```python
from build123d import *

# Parameters (mm, degrees)
F0_W     = 39.75
F0_H     = 5
F0_W_2   = 4
F0_H_2   = 9
F0_H_3   = 77
F0_W_3   = 3
F0_H_4   = 26.5
F0_H_5   = 1.95
F0_W_4   = 5
F0_H_6   = 17
F0_H_7   = 23.1
F1_DEPTH = 8


with BuildPart() as f1:
    # F0 (on Top) → F1 (new body)
    with BuildSketch(Plane.XY):
        Polygon((-32.4509056807, -49.8260023594), (-32.4509056807, -58.8260023594), (7.2990943193, -58.8260023594), (7.2990943193, -49.8260023594), (-26.0348562151, -49.8260023594), align=None)
        with Locations((-12.5759056807, -61.3260023594)):
            Rectangle(F0_W, F0_H)
        with Locations((9.2990943193, -54.3260023594)):
            Rectangle(F0_W_2, F0_H_2)
        Polygon((11.2990943193, -58.8260023594), (7.2990943193, -58.8260023594), (7.2990943193, -63.8260023594), (14.2990943193, -63.8260023594), (19.2990943193, -63.8260023594), (58.2990943193, -63.8260023594), (58.2990943193, -22.3260023594), (53.2990943193, -22.3260023594), (53.2990943193, -25.3760023594), (53.2990943193, -27.3260023594), (51.3490943193, -27.3260023594), (28.5490943193, -27.3260023594), (23.2990943193, -27.3260023594), (23.2990943193, -32.3260023594), (53.5990943193, -32.3260023594), (55.2990943193, -32.3260023594), (55.2990943193, -34.0260023594), (55.2990943193, -57.1260023594), (55.2990943193, -58.8260023594), (53.5990943193, -58.8260023594), (23.2990943193, -58.8260023594), (19.2990943193, -58.8260023594), (14.2990943193, -58.8260023594), align=None)
        with BuildLine():
            Line((-32.4509056807, -0.3260023594), (-32.4509056807, -49.8260023594))
            Line((-32.4509056807, -49.8260023594), (-26.0348562151, -49.8260023594))
            Line((-26.0348562151, -49.8260023594), (7.2990943193, -49.8260023594))
            Line((7.2990943193, -49.8260023594), (11.2990943193, -49.8260023594))
            Line((11.2990943193, -49.8260023594), (11.2990943193, -49.2260023594))
            ThreePointArc((11.2990943193, -49.2260023594), (9.2990943193, -47.2260023594), (11.2990943193, -45.2260023594))
            Line((11.2990943193, -45.2260023594), (11.2990943193, -0.3260023594))
            Line((11.2990943193, -0.3260023594), (-32.4509056807, -0.3260023594))
        make_face()
        with Locations((-12.5759056807, -102.3260023594)):
            Rectangle(F0_W, F0_H_3)
        with Locations((12.7990943193, -54.3260023594)):
            Rectangle(F0_W_3, F0_H_2)
        Polygon((14.2990943193, -49.8260023594), (14.2990943193, -58.8260023594), (19.2990943193, -58.8260023594), (19.2990943193, -32.3260023594), (23.2990943193, -32.3260023594), (23.2990943193, -27.3260023594), (19.2990943193, -27.3260023594), (19.2990943193, -25.3760023594), (19.2990943193, -2.2760023594), (19.2990943193, -0.3260023594), (14.2990943193, -0.3260023594), (14.2990943193, -27.3260023594), (14.2990943193, -32.3260023594), (14.2990943193, -47.2260023594), align=None)
        with BuildLine():
            Line((11.2990943193, -49.2260023594), (11.2990943193, -49.8260023594))
            Line((11.2990943193, -49.8260023594), (14.2990943193, -49.8260023594))
            Line((14.2990943193, -49.8260023594), (14.2990943193, -47.2260023594))
            Line((14.2990943193, -47.2260023594), (13.2990943193, -47.2260023594))
            ThreePointArc((13.2990943193, -47.2260023594), (12.7133078817, -48.6402159218), (11.2990943193, -49.2260023594))
        make_face()
        with BuildLine():
            Line((14.2990943193, -0.3260023594), (11.2990943193, -0.3260023594))
            Line((11.2990943193, -0.3260023594), (11.2990943193, -45.2260023594))
            ThreePointArc((11.2990943193, -45.2260023594), (12.7133078817, -45.811788797), (13.2990943193, -47.2260023594))
            Line((13.2990943193, -47.2260023594), (14.2990943193, -47.2260023594))
            Line((14.2990943193, -47.2260023594), (14.2990943193, -32.3260023594))
            Line((14.2990943193, -32.3260023594), (14.2990943193, -27.3260023594))
            Line((14.2990943193, -27.3260023594), (14.2990943193, -0.3260023594))
        make_face()
        with Locations((21.2990943193, -45.5760023594)):
            Rectangle(F0_W_2, F0_H_4)
        with BuildLine():
            Line((23.2990943193, -32.3260023594), (23.2990943193, -58.8260023594))
            Line((23.2990943193, -58.8260023594), (53.5990943193, -58.8260023594))
            Line((53.5990943193, -58.8260023594), (53.5990943193, -58.3260023594))
            ThreePointArc((53.5990943193, -58.3260023594), (52.7505661819, -56.277474222), (54.7990943193, -57.1260023594))
            Line((54.7990943193, -57.1260023594), (55.2990943193, -57.1260023594))
            Line((55.2990943193, -57.1260023594), (55.2990943193, -34.0260023594))
            Line((55.2990943193, -34.0260023594), (54.7990943193, -34.0260023594))
            ThreePointArc((54.7990943193, -34.0260023594), (52.7505661819, -34.8745304968), (53.5990943193, -32.8260023594))
            Line((53.5990943193, -32.8260023594), (53.5990943193, -32.3260023594))
            Line((53.5990943193, -32.3260023594), (23.2990943193, -32.3260023594))
        make_face()
        with Locations((21.2990943193, -1.3010023594)):
            Rectangle(F0_W_2, F0_H_5)
        with BuildLine():
            Line((53.5990943193, -58.3260023594), (53.5990943193, -58.8260023594))
            Line((53.5990943193, -58.8260023594), (55.2990943193, -58.8260023594))
            Line((55.2990943193, -58.8260023594), (55.2990943193, -57.1260023594))
            Line((55.2990943193, -57.1260023594), (54.7990943193, -57.1260023594))
            ThreePointArc((54.7990943193, -57.1260023594), (54.4476224568, -57.9745304968), (53.5990943193, -58.3260023594))
        make_face()
        with Locations((55.7990943193, -13.8260023594)):
            Rectangle(F0_W_4, F0_H_6)
        with BuildLine():
            Line((28.5490943193, -0.3260023594), (23.2990943193, -0.3260023594))
            Line((23.2990943193, -0.3260023594), (23.2990943193, -2.2760023594))
            Line((23.2990943193, -2.2760023594), (27.3990943193, -2.2760023594))
            ThreePointArc((27.3990943193, -2.2760023594), (27.735921521, -1.462829561), (28.5490943193, -1.1260023594))
            Line((28.5490943193, -1.1260023594), (28.5490943193, -0.3260023594))
        make_face()
        with Locations((21.2990943193, -13.8260023594)):
            Rectangle(F0_W_2, F0_H_7)
        with BuildLine():
            Line((55.2990943193, -32.3260023594), (53.5990943193, -32.3260023594))
            Line((53.5990943193, -32.3260023594), (53.5990943193, -32.8260023594))
            ThreePointArc((53.5990943193, -32.8260023594), (54.4476224568, -33.177474222), (54.7990943193, -34.0260023594))
            Line((54.7990943193, -34.0260023594), (55.2990943193, -34.0260023594))
            Line((55.2990943193, -34.0260023594), (55.2990943193, -32.3260023594))
        make_face()
        with BuildLine():
            Line((23.2990943193, -25.3760023594), (23.2990943193, -27.3260023594))
            Line((23.2990943193, -27.3260023594), (28.5490943193, -27.3260023594))
            Line((28.5490943193, -27.3260023594), (28.5490943193, -26.5260023594))
            ThreePointArc((28.5490943193, -26.5260023594), (27.735921521, -26.1891751578), (27.3990943193, -25.3760023594))
            Line((27.3990943193, -25.3760023594), (23.2990943193, -25.3760023594))
        make_face()
        with Locations((21.2990943193, -26.3510023594)):
            Rectangle(F0_W_2, F0_H_5)
        with BuildLine():
            Line((53.2990943193, -25.3760023594), (53.2990943193, -22.3260023594))
            Line((53.2990943193, -22.3260023594), (53.2990943193, -5.3260023594))
            Line((53.2990943193, -5.3260023594), (53.2990943193, -2.2760023594))
            Line((53.2990943193, -2.2760023594), (52.4990943193, -2.2760023594))
            ThreePointArc((52.4990943193, -2.2760023594), (50.535921521, -3.0891751578), (51.3490943193, -1.1260023594))
            Line((51.3490943193, -1.1260023594), (51.3490943193, -0.3260023594))
            Line((51.3490943193, -0.3260023594), (28.5490943193, -0.3260023594))
            Line((28.5490943193, -0.3260023594), (28.5490943193, -1.1260023594))
            ThreePointArc((28.5490943193, -1.1260023594), (29.3622671177, -1.462829561), (29.6990943193, -2.2760023594))
            ThreePointArc((29.6990943193, -2.2760023594), (28.5490943193, -3.4260023594), (27.3990943193, -2.2760023594))
            Line((27.3990943193, -2.2760023594), (23.2990943193, -2.2760023594))
            Line((23.2990943193, -2.2760023594), (23.2990943193, -25.3760023594))
            Line((23.2990943193, -25.3760023594), (27.3990943193, -25.3760023594))
            ThreePointArc((27.3990943193, -25.3760023594), (28.5490943193, -24.2260023594), (29.6990943193, -25.3760023594))
            ThreePointArc((29.6990943193, -25.3760023594), (29.3622671177, -26.1891751578), (28.5490943193, -26.5260023594))
            Line((28.5490943193, -26.5260023594), (28.5490943193, -27.3260023594))
            Line((28.5490943193, -27.3260023594), (51.3490943193, -27.3260023594))
            Line((51.3490943193, -27.3260023594), (51.3490943193, -26.5260023594))
            ThreePointArc((51.3490943193, -26.5260023594), (50.535921521, -24.562829561), (52.4990943193, -25.3760023594))
            Line((52.4990943193, -25.3760023594), (53.2990943193, -25.3760023594))
        make_face()
        Polygon((53.2990943193, -5.3260023594), (58.2990943193, -5.3260023594), (58.2990943193, -0.3260023594), (53.2990943193, -0.3260023594), (53.2990943193, -2.2760023594), align=None)
        with BuildLine():
            Line((53.2990943193, -27.3260023594), (53.2990943193, -25.3760023594))
            Line((53.2990943193, -25.3760023594), (52.4990943193, -25.3760023594))
            ThreePointArc((52.4990943193, -25.3760023594), (52.1622671177, -26.1891751578), (51.3490943193, -26.5260023594))
            Line((51.3490943193, -26.5260023594), (51.3490943193, -27.3260023594))
            Line((51.3490943193, -27.3260023594), (53.2990943193, -27.3260023594))
        make_face()
        with BuildLine():
            Line((53.2990943193, -0.3260023594), (51.3490943193, -0.3260023594))
            Line((51.3490943193, -0.3260023594), (51.3490943193, -1.1260023594))
            ThreePointArc((51.3490943193, -1.1260023594), (52.1622671177, -1.462829561), (52.4990943193, -2.2760023594))
            Line((52.4990943193, -2.2760023594), (53.2990943193, -2.2760023594))
            Line((53.2990943193, -2.2760023594), (53.2990943193, -0.3260023594))
        make_face()
    extrude(amount=F1_DEPTH)


solid = f1.part
```
Geometry: final body of the model. Coordinates: model frame, mm. A direction names the side the tool comes from. Give positions to 0.01 mm unless a question says otherwise; leave off trailing zeros. Order: outer loops, then holes, each group sorted by start corner. A loop starts at its lowest first (then second) coordinate and runs counter-clockwise, first axis right, second up. Notation, with made-up numbers: (79.25, 79.5) -> (112.25, 79.5) arc R11 ccw to (112.25, 88.5) -> close; hole circle Ø10 at (61, 69). An arc over 180 degrees is marked (long way). Write each question's results on one line, items separated by ' | '. Start each with the question number.
1) Set-up query: faces 1 (the flat face through (-13, -140.826, 4)), 2 (the flat face through (7.299, -103, 4)). Return all of +Z, -Z, +X, -X, +Y, -Y with unobstructed straight access to the full face (end or side cutting, diameter ignored); none if empty.
2) Line query: line 1 (Y direction, x = 28, z = 0.5); line 2 (Y direction, x = 14, z = 2.25); line 3 (X direction, y = -100.5, z = 6). Output: solid intervals per line, ascending. Write a range as from..to.
3) Section A-A (z = 6.25). Return loops of the section in (x, y).
4) Section B-B (x = 22.5). Return loops of the section in (y, z), then the cut area to 3 significant figures.
5) Section C-C (y = -115). Return loops of the section in (x, z).
6) First-contact query: pin 1 (2.5 mm diameter, centred on y = -115.5, z = 2, fed in from +X); pin 2 (1.5 mm diameter, centred on x = 36, z = 5.5, fed in from -Y); pin 3 (3 mm diameter, centred on x = 53.6, y = -34.03, fed in from -Z). Flat tips, straight axial feed; report the tip coordinate or a pass-through.
Calculated:
1) face 1: +Z, -Z, +X, -X, -Y | face 2: +Z, -Z, +X, -Y
2) line 1: -63.83..-26.39, -24.37..-3.29, -1.27..-0.33 | line 2: -63.83..-0.33 | line 3: -32.45..7.3
3) outline: (-32.45, -140.83) -> (7.3, -140.83) -> (7.3, -63.83) -> (58.3, -63.83) -> (58.3, -0.33) -> (-32.45, -0.33) -> close; hole circle Ø4 at (11.3, -47.23); hole circle Ø2.3 at (28.55, -25.38); hole circle Ø2.3 at (28.55, -2.28); hole circle Ø2.3 at (51.35, -25.38); hole circle Ø2.3 at (51.35, -2.28); hole circle Ø2.4 at (53.6, -57.13); hole circle Ø2.4 at (53.6, -34.03)
4) outline: (-63.83, 0) -> (-0.33, 0) -> (-0.33, 8) -> (-63.83, 8) -> close | area: 508 mm2
5) outline: (-32.45, 0) -> (7.3, 0) -> (7.3, 8) -> (-32.45, 8) -> close
6) pin 1: x = 7.3 | pin 2: y = -63.83 | pin 3: z = 0
